from build123d import *

# Parameters (mm, degrees)
BASE_FLANGE1_DEPTH         = 2
EDGE_FLANGE1_DEPTH         = 14
FILLET1_R                  = 2
SKETCH9_W                  = 37
SKETCH9_H                  = 15
BOSS_EXTRUDE1_DEPTH        = 2
FILLET2_R                  = 2
CUT_EXTRUDE1_DEPTH         = 2
FILLET3_R                  = 2
M2_5_CLEARANCE_HOLE1_D     = 2.9
M2_5_CLEARANCE_HOLE1_DEPTH = 2
M4_CLEARANCE_HOLE1_D       = 4.5
SKETCH15_R                 = 11.5
CUT_EXTRUDE2_DEPTH         = 10


# Sheet-metal steps are written as plain solids
with BuildPart() as part:
    # Sketch1 → Base-Flange1 (new body)
    with BuildSketch(Plane(origin=(0, 0, 0), x_dir=(1, 0, 0), z_dir=(0, 1, 0))):
        Polygon((-17.5, -17.5), (-32.5, -17.5), (-32.5, 9.5), (-18.5, 9.5), (-18.5, 7.5), (-17.5, 7.5), (-17.5, 8.5), (-17.5, 17.5), (17.5, 17.5), (17.5, 8.5), (17.5, 7.5), (18.5, 7.5), (18.5, 9.5), (32.5, 9.5), (32.5, -17.5), (17.5, -17.5), align=None)
    extrude(amount=-BASE_FLANGE1_DEPTH)

    # Edge-Flange1 section (across the edge) → Edge-Flange1 (add)
    with BuildSketch(Plane(origin=(-18.5, 0, -11.5), x_dir=(0, 0, 1), z_dir=(-1, 0, 0))):
        with BuildLine():
            Line((-2, 2), (-2, 43))
            Line((-2, 43), (0, 43))
            Line((0, 43), (0, 2))
            ThreePointArc((0, 2), (0.585786438, 0.585786438), (2, 0))
            Line((2, 0), (2, -2))
            ThreePointArc((2, -2), (-0.828427125, -0.828427125), (-2, 2))
        make_face()
    edge_flange1 = extrude(amount=EDGE_FLANGE1_DEPTH)

    # Mirror1: Edge-Flange1 across plane
    add(edge_flange1.mirror(Plane(origin=(0, 0, 0), x_dir=(0, 0, 1), z_dir=(1, 0, 0))))

    # Fillet1
    fillet1_edges = [part.edges().sort_by_distance(p)[0] for p in [
        (-17.5, -1, -17.5),
        (17.5, -1, -17.5),
    ]]
    fillet(fillet1_edges, radius=FILLET1_R)

    # Sketch9 → Boss-Extrude1 (add)
    with BuildSketch(Plane.XY.offset(-11.5)):
        with Locations((0, 35.5)):
            Rectangle(SKETCH9_W, SKETCH9_H)
    extrude(amount=-BOSS_EXTRUDE1_DEPTH)

    # Fillet2
    fillet2_edges = [part.edges().sort_by_distance(p)[0] for p in [
        (-18.5, 28, -12.5),
        (18.5, 28, -12.5),
        (-32.5, 43, -12.5),
        (32.5, 43, -12.5),
    ]]
    fillet(fillet2_edges, radius=FILLET2_R)

    # Sketch10 → Cut-Extrude1 (cut)
    with BuildSketch(Plane(origin=(0, 0, 0), x_dir=(1, 0, 0), z_dir=(0, 1, 0))):
        Polygon((-32.5, 4.5), (-17.5, -17.5), (-32.5, -17.5), align=None)
    cut_extrude1 = extrude(amount=-CUT_EXTRUDE1_DEPTH, mode=Mode.SUBTRACT)

    # Mirror2: Cut-Extrude1 across plane
    add(cut_extrude1.mirror(Plane(origin=(0, 0, 0), x_dir=(0, 0, 1), z_dir=(1, 0, 0))), mode=Mode.SUBTRACT)

    # Fillet3
    fillet3_edges = [part.edges().sort_by_distance(p)[0] for p in [
        (-32.5, -1, -4.5),
        (-17.5, -1, 17.5),
        (32.5, -1, -4.5),
        (17.5, -1, 17.5),
    ]]
    fillet(fillet3_edges, radius=FILLET3_R)

    # M2.5 Clearance Hole1
    with Locations(Plane(origin=(0, 0, 0), x_dir=(1, 0, 0), z_dir=(0, 1, 0))):
        with Locations((13, -13), (-13, -13), (-13, 13), (13, 13)):
            Hole(M2_5_CLEARANCE_HOLE1_D / 2, depth=M2_5_CLEARANCE_HOLE1_DEPTH)

    # M4 Clearance Hole1 (through all)
    with Locations(Plane.XY.offset(-11.5)):
        with Locations((-25.5, 33), (25.5, 33)):
            Hole(M4_CLEARANCE_HOLE1_D / 2)

    # Sketch15 → Cut-Extrude2 (cut)
    with BuildSketch(Plane(origin=(0, 0, 0), x_dir=(1, 0, 0), z_dir=(0, 1, 0))):
        with Locations(Location((0, 0, 0), (0, 0, 270))):
            Circle(SKETCH15_R)
    extrude(amount=-CUT_EXTRUDE2_DEPTH, mode=Mode.SUBTRACT)


solid = part.part
Geometry check sheet. Reference: the model listing, model coordinates, mm. A direction names the side the tool comes from. Round coordinates to 2 decimals unless told otherwise and drop trailing zeros. Write each loop counter-clockwise with the first axis right and the second up, starting at its lowest first coordinate (ties: lowest second). Pieces come first, ordered by that corner, then holes. Notation, with made-up numbers: (41.5, 51.25) -> (96.5, 51.25) arc R34 ccw to (96.5, 86.25) -> close; hole circle Ø1 at (55.5, 34). An arc over 180 degrees is marked (long way). One line per item, written item: value. Start each with the question number.
(1) Draft check along Y on faces 5 (the flat face through (0, -2, -12)), 6 (the cylindrical face through (24.29, 34.897, -12.514)), 7 (the cylindrical face through (-25.4, 0.6, -10.93)), 8 (the cylindrical face through (-17.39, -1.01, 17.26)). Enter one of: +Y half, -Y half, draft (parallel to the pull), parting line (faces both ways), or undercut.
(2) Go/stop test with flat-tipped pins: pin 1 Ø1.5 at (x, z) = (-2.5, -9) entering from -Y; pin 2 Ø3.5 at (x, z) = (13, 13) entering from +Y; pin 3 Ø0.5 at (x, y) = (-18, -0.5) entering from -Z; pin 4 Ø0.6 at (y, z) = (-1, -13) entering from +X. Record where each tip stops, or that it passes through.
(3) Cross-section at C-C, the plane y = 33. Record the cut outline in (x, z).
(4) Cross-section at A-A, the plane x = 0. Record the cut outline in (y, z).
(5) Cross-section at B-B, the plane y = 23. Record the cut outline in (x, z).
(6) Scan lines: line 1 (Z direction, x = 13, y = -1); line 2 (Y direction, x = -21, z = 3.5); line 3 (X direction, y = 35, z = -13). Record each from-to range of solid material in increasing order. Write a range as [from, to].
(7) Access from +Z, -Z, +X, -X, +Y, -Y to the whole of each face (thin tool, end or side, straight path). Record for faces 1 (the flat face through (0, 32, -11.5)), 2 (the cylindrical face through (14.15, -1.01, -12.12)), 3 (the cylindrical face through (-17.9, 27.43, -12.51)), 4 (the cylindrical face through (25.402, -0.859, -12.297)).
(8) Cross-section at D-D, the plane z = 0. Record the cut outline in (x, y), and give its area (3 significant figures).
Answer:
1. face 5: -Y half
1. face 6: undercut
1. face 7: +Y half
1. face 8: draft
2. pin 1: through
2. pin 2: y = 0
2. pin 3: z = -7.5
2. pin 4: x = 17.5
3. outline: (-32.5, -13.5) -> (-27.75, -13.5) -> (-27.75, -11.5) -> (-32.5, -11.5) -> close; (-23.25, -13.5) -> (23.25, -13.5) -> (23.25, -11.5) -> (-23.25, -11.5) -> close; (27.75, -13.5) -> (32.5, -13.5) -> (32.5, -11.5) -> (27.75, -11.5) -> close
4. outline: (-2, -17.5) -> (0, -17.5) -> (0, -11.5) -> (-2, -11.5) -> close; (-2, 11.5) -> (0, 11.5) -> (0, 17.5) -> (-2, 17.5) -> close; (28, -13.5) -> (43, -13.5) -> (43, -11.5) -> (28, -11.5) -> close
5. outline: (-32.5, -13.5) -> (-18.5, -13.5) -> (-18.5, -11.5) -> (-32.5, -11.5) -> close; (18.5, -13.5) -> (32.5, -13.5) -> (32.5, -11.5) -> (18.5, -11.5) -> close
6. line 1: [-17.5, -14.45], [-11.55, 11.55], [14.45, 17.5]
6. line 2: [-2, 0]
6. line 3: [-32.5, -26.53], [-24.47, 24.47], [26.53, 32.5]
7. face 1: +Z, +X, -X, +Y
7. face 2: -Y
7. face 3: +Z, -Z
7. face 4: -Z, +X, -Y
8. outline: (-29.43, -2) -> (-11.5, -2) -> (-11.5, 0) -> (-29.43, 0) -> close; (11.5, -2) -> (29.43, -2) -> (29.43, 0) -> (11.5, 0) -> close
8. area: 71.7 mm²
